Source: three-view drawing plus pictorial views. Frame: mm from the lowest corner of the part. A direction names the side the tool comes from. Give positions to 0.01 mm unless a question says otherwise; leave off trailing zeros. Order: outer loops, then holes, each group sorted by start corner. A loop starts at its lowest first (then second) coordinate and runs counter-clockwise, first axis right, second up. Notation, with made-up numbers: (34.5, -39.5) -> (93.5, -39.5) arc R20 cw to (93.5, -26.5) -> close; hole circle Ø8 at (47, -20.5). An arc over 180 degrees is marked (long way). Use a Markdown table: item, result. Add a question column.
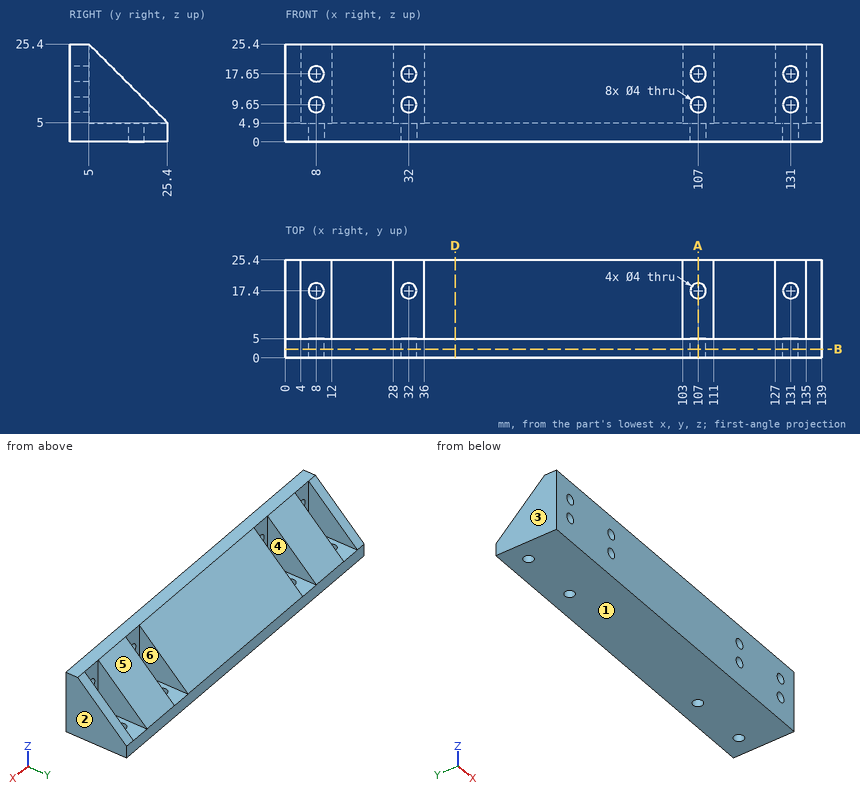
Q1. Access query for the marked faces 5 and 6. Directions: +Z, -Z, +X, -X, +Y, -Y. A direction counts if a zero-diameter tool reaches every point of the face in a straight line with its end or side. Return the directions, or none.
Q2. First-contact query: pin 1 (4 mm diameter, centred on x = 107, z = 18.5, fed in from +Y); pin 2 (5 mm diameter, centred on x = 107, y = 17.4, fed in from +Z); pin 3 (9 mm diameter, centred on x = 32, y = 12, fed in from +Z). Flat tips, straight axial feed; report the tip coordinate or a pass-through.
Q3. Section query D-D (x = 44). Return loops of the section in (y, z), plus the area to 3 significant figures.
Q4. Section query A-A (x = 107). Return loops of the section in (y, z), plus the area to 3 significant figures.
Q5. Section query B-B (y = 2.25). Give the number of separate pieces and of enclosed holes in the cut face, plus the area to 3 significant figures.
Q6. Ray query, line 1 (X direction, y = 9.75, z = 8.5); line 2 (Z direction, x = 131, y = 1.7); line 3 (X direction, y = 1.4, z = 9.65). Return the intervals inside material, ascending.
Q7. Draft query along X for the marked faces 1, 2, 3 and 4. Return one class per face: +X half, -X half, draft (parallel to the pull), parting line (faces both ways), or undercut.
Solution:
| question | item | result |
|---|---|---|
| 1 | face 5 | +Z, +X, -X, +Y |
| 1 | face 6 | +Z, +Y |
| 2 | pin 1 | stops at y = 5 |
| 2 | pin 2 | stops at z = 4.9 |
| 2 | pin 3 | stops at z = 20.46 |
| 3 | outline | (0, 0) -> (25.4, 0) -> (25.4, 5) -> (5, 25.4) -> (0, 25.4) -> close |
| 3 | area | 437 mm² |
| 4 | outline | (0, 0) -> (15.4, 0) -> (15.4, 4.9) -> (5, 4.9) -> (5, 7.65) -> (0, 7.65) -> close; (0, 11.65) -> (5, 11.65) -> (5, 15.65) -> (0, 15.65) -> close; (0, 19.65) -> (5, 19.65) -> (5, 25.4) -> (0, 25.4) -> close; (19.4, 0) -> (25.4, 0) -> (25.4, 4.9) -> (19.4, 4.9) -> close |
| 4 | area | 167 mm² |
| 5 | separate pieces | 1 |
| 5 | enclosed holes | 8 |
| 5 | area | 3,430 mm² |
| 6 | line 1 | x = 0 to 4, 12 to 28, 36 to 103, 111 to 127, 135 to 139 |
| 6 | line 2 | z = 0 to 7.65, 11.65 to 15.65, 19.65 to 25.4 |
| 6 | line 3 | x = 0 to 6, 10 to 30, 34 to 105, 109 to 129, 133 to 139 |
| 7 | face 1 | draft |
| 7 | face 2 | +X half |
| 7 | face 3 | -X half |
| 7 | face 4 | undercut |
